Part model, mm, in its own coordinate system. A direction names the side the tool comes from. Coordinates: 2 decimals unless noted, no trailing zeros. Order: outer loops, then holes, each group sorted by start corner. A loop starts at its lowest first (then second) coordinate and runs counter-clockwise, first axis right, second up. Notation, with made-up numbers: (11.25, 5.5) - (67.25, 5.5) arc R24 ccw to (67.25, 22.5) - close; hole circle Ø7 at (-32.75, 89). An arc over 180 degrees is marked (long way). Use a Markdown table: item, result. Add a question column.
1) Wall check: L1, parallel to X at y = 6.25, z = -105.5; L2, parallel to X at y = 3, z = -55.5; L3, parallel to Z at x = 316.5, y = 5.5 (3 decimals). Give the ranges that are in metal, low to high. Write a range as [from, to].
2) Saw through at B-B on y = 5.25. Count the separate pieces of the cut face and the enclosed holes in it, then the cut area to 3 significant figures.
3) Saw through at A-A on x = 326. List the corners of the cut face in (y, z) (3 decimals), then the cut area to 3 significant figures.
4) Drop a flat-ended pin along its axis: P1, Ø10, axis at x = 228.5, z = -123.5, coming from the -Y side. Give the stop position or say it passes through.
5) Two-plate mould, pull along X, no slides. Class faces 1 (the face through (0, 3, -74)), 2 (the face through (254, 3, -74)), 3 (the face through (188, 0, -76)): +X half, -X half, draft (parallel to the pull), parting line (faces both ways), or undercut.
6) Tool access for faces 4 (the face through (188, 6.35, -76)), 5 (the face through (306, 3, -98.425)): list every direction of +Z, -Z, +X, -X, +Y, -Y with a clear straight run to the whole face (end or side of a thin tool).
```python
from build123d import *

# Parameters (mm, degrees)
SKETCH1_W           = 381
SKETCH1_H           = 149.225
BOSS_EXTRUDE1_DEPTH = 6.35
SKETCH9_W           = 19.05
SKETCH9_H           = 14.2875
CUT_EXTRUDE1_DEPTH  = 7.62


with BuildPart() as part:
    # Sketch1 → Boss-Extrude1 (new body)
    with BuildSketch(Plane(origin=(0, 0, 0), x_dir=(1, 0, 0), z_dir=(0, 1, 0))):
        with Locations((190.5, 74.6125)):
            Rectangle(SKETCH1_W, SKETCH1_H)
        with BuildLine():
            Line((342.9, 95.25), (342.9, 53.975))
            ThreePointArc((342.9, 53.975), (341.97006403, 51.72993597), (339.725, 50.8))
            Line((339.725, 50.8), (257.175, 50.8))
            ThreePointArc((257.175, 50.8), (254.92993597, 51.72993597), (254, 53.975))
            Line((254, 53.975), (254, 95.25))
            ThreePointArc((254, 95.25), (254.92993597, 97.49506403), (257.175, 98.425))
            Line((257.175, 98.425), (339.725, 98.425))
            ThreePointArc((339.725, 98.425), (341.97006403, 97.49506403), (342.9, 95.25))
        make_face(mode=Mode.SUBTRACT)
        with BuildLine():
            Line((41.275, 98.425), (123.825, 98.425))
            ThreePointArc((123.825, 98.425), (126.07006403, 97.49506403), (127, 95.25))
            Line((127, 95.25), (127, 53.975))
            ThreePointArc((127, 53.975), (126.07006403, 51.72993597), (123.825, 50.8))
            Line((123.825, 50.8), (41.275, 50.8))
            ThreePointArc((41.275, 50.8), (39.02993597, 51.72993597), (38.1, 53.975))
            Line((38.1, 53.975), (38.1, 95.25))
            ThreePointArc((38.1, 95.25), (39.02993597, 97.49506403), (41.275, 98.425))
        make_face(mode=Mode.SUBTRACT)
    extrude(amount=BOSS_EXTRUDE1_DEPTH)

    # Sketch9 → Cut-Extrude1 (cut)
    with BuildSketch(Plane(origin=(0, 6.35, 0), x_dir=(1, 0, 0), z_dir=(0, 1, 0))):
        with Locations((117.475, 102.39375)):
            Rectangle(SKETCH9_W, SKETCH9_H)
        with Locations((117.475, 46.83125)):
            Rectangle(SKETCH9_W, SKETCH9_H)
        with Locations((263.525, 46.83125)):
            Rectangle(SKETCH9_W, SKETCH9_H)
        with Locations((263.525, 102.39375)):
            Rectangle(SKETCH9_W, SKETCH9_H)
    extrude(amount=-CUT_EXTRUDE1_DEPTH, mode=Mode.SUBTRACT)


solid = part.part
```
Results are:
| question | item | result |
|---|---|---|
| 1 | L1 | [0, 107.95], [127, 254], [273.05, 381] |
| 1 | L2 | [0, 38.1], [127, 254], [342.9, 381] |
| 1 | L3 | [-149.225, -98.425], [-50.8, 0] |
| 2 | separate pieces | 1 |
| 2 | enclosed holes | 2 |
| 2 | area | 47,500 mm2 |
| 3 | outline | (0, -149.225) - (6.35, -149.225) - (6.35, -98.425) - (0, -98.425) - close; (0, -50.8) - (6.35, -50.8) - (6.35, 0) - (0, 0) - close |
| 3 | area | 645 mm2 |
| 4 | P1 | y = 0 |
| 5 | face 1 | -X half |
| 5 | face 2 | undercut |
| 5 | face 3 | draft |
| 6 | face 4 | +Z, -Z, +X, -X, +Y |
| 6 | face 5 | +Y, -Y |
